Could you check a few things on this model? Use its own coordinates, in mm. Coordinates: 2 decimals unless noted, no trailing zeros. Write each loop counter-clockwise with the first axis right and the second up, starting at its lowest first coordinate (ties: lowest second). Pieces come first, ordered by that corner, then holes.
```python
from build123d import *

# Parameters (mm, degrees)
BOSS_EXTRUDE1_DEPTH = 6.35
FILLET1_R           = 9.525
SKETCH2_R           = 1.5
CUT_EXTRUDE1_DEPTH  = 173.855351378
LPATTERN1_COUNT     = 2
LPATTERN1_PITCH     = 77.47


with BuildPart() as part:
    # Sketch1 → Boss-Extrude1 (new body)
    with BuildSketch(Plane(origin=(0, 0, 0), x_dir=(1, 0, 0), z_dir=(0, 1, 0))):
        Polygon((-120.65, -101.6), (-120.65, 82.55), (120.65, 82.55), (120.65, -101.6), (139.7, -101.6), (139.7, 101.6), (-139.7, 101.6), (-139.7, -101.6), align=None)
    extrude(amount=-BOSS_EXTRUDE1_DEPTH)

    # Fillet1
    fillet1_edges = [part.edges().sort_by_distance(p)[0] for p in [
        (120.65, -3.175, -82.55),
        (-120.65, -3.175, -82.55),
    ]]
    fillet(fillet1_edges, radius=FILLET1_R)

    # Sketch2 → Cut-Extrude1 (cut, through all)
    with BuildSketch(Plane(origin=(0, 0, 0), x_dir=(1, 0, 0), z_dir=(0, 1, 0))):
        with Locations(Location((-133.35, -88.9, 0), (0, 0, 270))):
            Circle(SKETCH2_R)
        with Locations(Location((-127, -95.25, 0), (0, 0, 270))):
            Circle(SKETCH2_R)
        with Locations(Location((133.35, -88.9, 0), (0, 0, 90))):
            Circle(SKETCH2_R)
        with Locations(Location((127, -95.25, 0), (0, 0, 90))):
            Circle(SKETCH2_R)
        with Locations(Location((132.42006403, 94.32006403, 0), (0, 0, 270))):
            Circle(SKETCH2_R)
        with Locations(Location((125.140128061, 87.040128061, 0), (0, 0, 270))):
            Circle(SKETCH2_R)
        with Locations(Location((-125.140128061, 87.040128061, 0), (0, 0, 90))):
            Circle(SKETCH2_R)
        with Locations(Location((-132.42006403, 94.32006403, 0), (0, 0, 90))):
            Circle(SKETCH2_R)
    cut_extrude1 = extrude(amount=-CUT_EXTRUDE1_DEPTH, mode=Mode.SUBTRACT)

    # LPattern1: Cut-Extrude1 ×2
    with Locations(*[(0, 0, -i * LPATTERN1_PITCH) for i in range(1, LPATTERN1_COUNT)]):
        add(cut_extrude1, mode=Mode.SUBTRACT)


solid = part.part
```
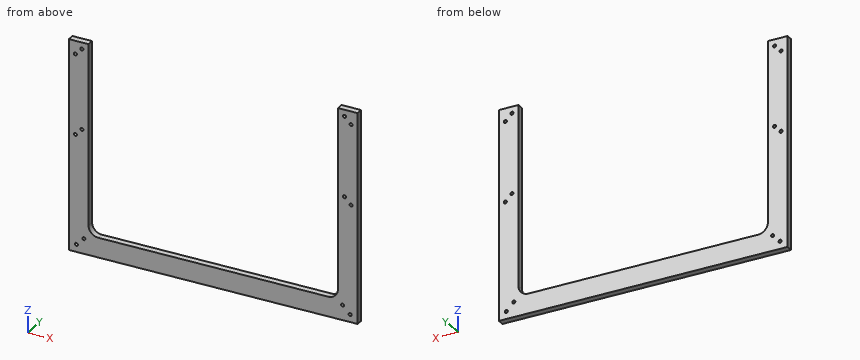
Item 1: I want a section at A-A, the plane z = 5. List the corners of the cut face in (x, y) for me.
Item 2: I want a section at C-C, the plane x = 103.5. List the corners of the cut face in (y, z) for me, then the cut area to 3 significant figures.
Item 3: If I drill on line 1 along X through (y, z) = (-2.75, 11.43); line 2 along X through (y, z) = (-3.5, 17.78); line 3 along X through (y, z) = (-2.25, 41), over which ranges is the centre line in solid material (lowest first)?
Item 4: Will these pins go through, and if not, where does the flat tip stop? pin 1 Ø3 at (x, y) = (35, -4.5) entering from +Z; pin 2 Ø2.5 at (x, z) = (-133.35, 88.9) entering from -Y; pin 3 Ø4 at (x, z) = (127, 95.25) entering from +Y.
Item 5: I want a section at B-B, the plane y = -4.25. Count the separate pieces of the cut face and the enclosed holes in it, then the cut area to 3 significant figures.
Taken from the geometry:
1. outline: (-139.7, -6.35) - (-120.65, -6.35) - (-120.65, 0) - (-139.7, 0) - close; (120.65, -6.35) - (139.7, -6.35) - (139.7, 0) - (120.65, 0) - close
2. outline: (-6.35, -101.6) - (0, -101.6) - (0, -82.55) - (-6.35, -82.55) - close
2. area: 121 mm2
3. line 1: x = -139.7 to -134.85, -131.85 to -120.65, 120.65 to 131.85, 134.85 to 139.7
3. line 2: x = -139.7 to -128.5, -125.5 to -120.65, 120.65 to 125.5, 128.5 to 139.7
3. line 3: x = -139.7 to -120.65, 120.65 to 139.7
4. pin 1: stops at z = -82.55
4. pin 2: passes through
4. pin 3: stops at y = 0
5. separate pieces: 1
5. enclosed holes: 12
5. area: 12,300 mm2
